Part model, mm, in its own coordinate system. A direction names the side the tool comes from. Give positions to 0.01 mm unless a question says otherwise; leave off trailing zeros. Write each loop counter-clockwise with the first axis right and the second up, starting at its lowest first coordinate (ties: lowest second). Pieces come first, ordered by that corner, then holes. Notation, with made-up numbers: (52, 4.25) - (73, 4.25) arc R20 ccw to (73, 40.25) - close; hole circle Ø8 at (44.25, 29.25). An arc over 180 degrees is marked (long way). Answer in a Markdown table with one row per item. Add a question column.
1. Band-saw the part on B-B on x = 24.5. Write the cut outline in (y, z), plus the area to 3 significant figures.
2. Band-saw the part on D-D on x = 0. Write the cut outline in (y, z), plus the area to 4 significant figures.
3. Band-saw the part on A-A on z = 5. Write the cut outline in (x, y).
4. Probe line 1 along X through (y, z) = (10.75, 5); line 2 along Y through (x, z) = (-7.5, 85.5); line 3 along X through (y, z) = (8.5, 65). List the from-to ranges inside material, lowest first.
5. Band-saw the part on C-C on y = -6.5. Write the cut outline in (x, z).
6. Which spindle directions (+Z, -Z, +X, -X, +Y, -Y) get a long thin tool onto all of the face, cutting with end or side? Do faces 5 (the flat face through (19, -1, 54)), 6 (the cylindrical face through (-15.58, -12.39, 54.23)). Say none if no direction does.
7. Drop flat-ended pins along their axis: pin 1 Ø3.5 at (x, z) = (24.5, 25) entering from -Y; pin 2 Ø3.5 at (x, z) = (-23.5, 62.5) entering from -Y; pin 3 Ø10 at (x, z) = (21, 52) entering from -Y; pin 4 Ø1 at (x, z) = (-13, 50) entering from -Y. Give the stop position or say it passes through.
8. Pull direction Z, two halves, no side cores. Call faces 1 (the cylindrical face through (24, 9, 103)), 2 (the flat face through (-25, 3, 54)), 3 (the flat face through (0, 11, 110)), 4 (the cylindrical face through (-25, 9, 43)): released by +Z, released by -Z, zero draft, split by the parting line, or undercut.
```python
from build123d import *

# Parameters (mm, degrees)
CROQUIS1_R              = 10.25
SALIENTE_EXTRUIR1_DEPTH = 110
CORTAR_EXTRUIR1_REACH   = 117.59
CROQUIS2_R              = 2.06


with BuildPart() as part:
    # Croquis1 → Saliente-Extruir1 (new body)
    with BuildSketch(Plane.XY):
        with BuildLine():
            Line((30, 16), (-30, 16))
            Line((-30, 16), (-30, 3))
            Line((-30, 3), (-19, 3))
            Line((-19, 3), (-19, -4))
            ThreePointArc((-19, -4), (-15.485281374, -12.485281374), (-7, -16))
            Line((-7, -16), (7, -16))
            ThreePointArc((7, -16), (15.485281374, -12.485281374), (19, -4))
            Line((19, -4), (19, 3))
            Line((19, 3), (30, 3))
            Line((30, 3), (30, 16))
        make_face()
        Circle(CROQUIS1_R, mode=Mode.SUBTRACT)
    extrude(amount=SALIENTE_EXTRUIR1_DEPTH)

    # Croquis2 → Cortar-Extruir1 (cut, up to next)
    with BuildSketch(Plane.XZ.offset(-3), mode=Mode.PRIVATE) as cortar_extruir1_sk1:
        with Locations(Location((-24.5, 105, 0), (0, 0, 270))):
            Circle(CROQUIS2_R)
    cortar_extruir1_tool1 = extrude(cortar_extruir1_sk1.sketch, amount=-CORTAR_EXTRUIR1_REACH, mode=Mode.PRIVATE) & part.part
    # Croquis2 → Cortar-Extruir1 (cut, up to next)
    with BuildSketch(Plane.XZ.offset(-3), mode=Mode.PRIVATE) as cortar_extruir1_sk2:
        with Locations(Location((-24.5, 85, 0), (0, 0, 270))):
            Circle(CROQUIS2_R)
    cortar_extruir1_tool2 = extrude(cortar_extruir1_sk2.sketch, amount=-CORTAR_EXTRUIR1_REACH, mode=Mode.PRIVATE) & part.part
    # Croquis2 → Cortar-Extruir1 (cut, up to next)
    with BuildSketch(Plane.XZ.offset(-3), mode=Mode.PRIVATE) as cortar_extruir1_sk3:
        with Locations(Location((-24.5, 65, 0), (0, 0, 270))):
            Circle(CROQUIS2_R)
    cortar_extruir1_tool3 = extrude(cortar_extruir1_sk3.sketch, amount=-CORTAR_EXTRUIR1_REACH, mode=Mode.PRIVATE) & part.part
    # Croquis2 → Cortar-Extruir1 (cut, up to next)
    with BuildSketch(Plane.XZ.offset(-3), mode=Mode.PRIVATE) as cortar_extruir1_sk4:
        with Locations(Location((-24.5, 45, 0), (0, 0, 270))):
            Circle(CROQUIS2_R)
    cortar_extruir1_tool4 = extrude(cortar_extruir1_sk4.sketch, amount=-CORTAR_EXTRUIR1_REACH, mode=Mode.PRIVATE) & part.part
    # Croquis2 → Cortar-Extruir1 (cut, up to next)
    with BuildSketch(Plane.XZ.offset(-3), mode=Mode.PRIVATE) as cortar_extruir1_sk5:
        with Locations(Location((-24.5, 25, 0), (0, 0, 270))):
            Circle(CROQUIS2_R)
    cortar_extruir1_tool5 = extrude(cortar_extruir1_sk5.sketch, amount=-CORTAR_EXTRUIR1_REACH, mode=Mode.PRIVATE) & part.part
    # Croquis2 → Cortar-Extruir1 (cut, up to next)
    with BuildSketch(Plane.XZ.offset(-3), mode=Mode.PRIVATE) as cortar_extruir1_sk6:
        with Locations(Location((-24.5, 5, 0), (0, 0, 270))):
            Circle(CROQUIS2_R)
    cortar_extruir1_tool6 = extrude(cortar_extruir1_sk6.sketch, amount=-CORTAR_EXTRUIR1_REACH, mode=Mode.PRIVATE) & part.part
    # Croquis2 → Cortar-Extruir1 (cut, up to next)
    with BuildSketch(Plane.XZ.offset(-3), mode=Mode.PRIVATE) as cortar_extruir1_sk7:
        with Locations(Location((24.5, 5, 0), (0, 0, 270))):
            Circle(CROQUIS2_R)
    cortar_extruir1_tool7 = extrude(cortar_extruir1_sk7.sketch, amount=-CORTAR_EXTRUIR1_REACH, mode=Mode.PRIVATE) & part.part
    # Croquis2 → Cortar-Extruir1 (cut, up to next)
    with BuildSketch(Plane.XZ.offset(-3), mode=Mode.PRIVATE) as cortar_extruir1_sk8:
        with Locations(Location((24.5, 25, 0), (0, 0, 270))):
            Circle(CROQUIS2_R)
    cortar_extruir1_tool8 = extrude(cortar_extruir1_sk8.sketch, amount=-CORTAR_EXTRUIR1_REACH, mode=Mode.PRIVATE) & part.part
    # Croquis2 → Cortar-Extruir1 (cut, up to next)
    with BuildSketch(Plane.XZ.offset(-3), mode=Mode.PRIVATE) as cortar_extruir1_sk9:
        with Locations(Location((24.5, 45, 0), (0, 0, 270))):
            Circle(CROQUIS2_R)
    cortar_extruir1_tool9 = extrude(cortar_extruir1_sk9.sketch, amount=-CORTAR_EXTRUIR1_REACH, mode=Mode.PRIVATE) & part.part
    # Croquis2 → Cortar-Extruir1 (cut, up to next)
    with BuildSketch(Plane.XZ.offset(-3), mode=Mode.PRIVATE) as cortar_extruir1_sk10:
        with Locations(Location((24.5, 65, 0), (0, 0, 270))):
            Circle(CROQUIS2_R)
    cortar_extruir1_tool10 = extrude(cortar_extruir1_sk10.sketch, amount=-CORTAR_EXTRUIR1_REACH, mode=Mode.PRIVATE) & part.part
    # Croquis2 → Cortar-Extruir1 (cut, up to next)
    with BuildSketch(Plane.XZ.offset(-3), mode=Mode.PRIVATE) as cortar_extruir1_sk11:
        with Locations(Location((24.5, 85, 0), (0, 0, 270))):
            Circle(CROQUIS2_R)
    cortar_extruir1_tool11 = extrude(cortar_extruir1_sk11.sketch, amount=-CORTAR_EXTRUIR1_REACH, mode=Mode.PRIVATE) & part.part
    # Croquis2 → Cortar-Extruir1 (cut, up to next)
    with BuildSketch(Plane.XZ.offset(-3), mode=Mode.PRIVATE) as cortar_extruir1_sk12:
        with Locations(Location((24.5, 105, 0), (0, 0, 270))):
            Circle(CROQUIS2_R)
    cortar_extruir1_tool12 = extrude(cortar_extruir1_sk12.sketch, amount=-CORTAR_EXTRUIR1_REACH, mode=Mode.PRIVATE) & part.part
    add(cortar_extruir1_tool1.solids().sort_by_distance((-24.5, 3, 105))[0], mode=Mode.SUBTRACT)
    add(cortar_extruir1_tool2.solids().sort_by_distance((-24.5, 3, 85))[0], mode=Mode.SUBTRACT)
    add(cortar_extruir1_tool3.solids().sort_by_distance((-24.5, 3, 65))[0], mode=Mode.SUBTRACT)
    add(cortar_extruir1_tool4.solids().sort_by_distance((-24.5, 3, 45))[0], mode=Mode.SUBTRACT)
    add(cortar_extruir1_tool5.solids().sort_by_distance((-24.5, 3, 25))[0], mode=Mode.SUBTRACT)
    add(cortar_extruir1_tool6.solids().sort_by_distance((-24.5, 3, 5))[0], mode=Mode.SUBTRACT)
    add(cortar_extruir1_tool7.solids().sort_by_distance((24.5, 3, 5))[0], mode=Mode.SUBTRACT)
    add(cortar_extruir1_tool8.solids().sort_by_distance((24.5, 3, 25))[0], mode=Mode.SUBTRACT)
    add(cortar_extruir1_tool9.solids().sort_by_distance((24.5, 3, 45))[0], mode=Mode.SUBTRACT)
    add(cortar_extruir1_tool10.solids().sort_by_distance((24.5, 3, 65))[0], mode=Mode.SUBTRACT)
    add(cortar_extruir1_tool11.solids().sort_by_distance((24.5, 3, 85))[0], mode=Mode.SUBTRACT)
    add(cortar_extruir1_tool12.solids().sort_by_distance((24.5, 3, 105))[0], mode=Mode.SUBTRACT)


solid = part.part
```
Values:
| question | item | result |
|---|---|---|
| 1 | outline | (3, 0) - (16, 0) - (16, 2.94) - (3, 2.94) - close; (3, 7.06) - (16, 7.06) - (16, 22.94) - (3, 22.94) - close; (3, 27.06) - (16, 27.06) - (16, 42.94) - (3, 42.94) - close; (3, 47.06) - (16, 47.06) - (16, 62.94) - (3, 62.94) - close; (3, 67.06) - (16, 67.06) - (16, 82.94) - (3, 82.94) - close; (3, 87.06) - (16, 87.06) - (16, 102.94) - (3, 102.94) - close; (3, 107.06) - (16, 107.06) - (16, 110) - (3, 110) - close |
| 1 | area | 1,110 mm² |
| 2 | outline | (-16, 0) - (-10.25, 0) - (-10.25, 110) - (-16, 110) - close; (10.25, 0) - (16, 0) - (16, 110) - (10.25, 110) - close |
| 2 | area | 1,265 mm² |
| 3 | outline | (-30, 3) - (-26.56, 3) - (-26.56, 16) - (-30, 16) - close; (-22.44, 3) - (-19, 3) - (-19, -4) arc R12 ccw to (-7, -16) - (7, -16) arc R12 ccw to (19, -4) - (19, 3) - (22.44, 3) - (22.44, 16) - (-22.44, 16) - close; (26.56, 3) - (30, 3) - (30, 16) - (26.56, 16) - close; hole circle Ø20.5 at (0, 0) |
| 4 | line 1 | x = -30 to -26.56, -22.44 to 22.44, 26.56 to 30 |
| 4 | line 2 | y = -15.99 to -6.99, 6.99 to 16 |
| 4 | line 3 | x = -30 to -26.56, -22.44 to -5.73, 5.73 to 22.44, 26.56 to 30 |
| 5 | outline | (-18.74, 0) - (-7.93, 0) - (-7.93, 110) - (-18.74, 110) - close; (7.93, 0) - (18.74, 0) - (18.74, 110) - (7.93, 110) - close |
| 6 | face 5 | +Z, -Z, +X, -Y |
| 6 | face 6 | +Z, -Z, -X, -Y |
| 7 | pin 1 | passes through |
| 7 | pin 2 | stops at y = 3 |
| 7 | pin 3 | stops at y = -11.94 |
| 7 | pin 4 | stops at y = -14.67 |
| 8 | face 1 | undercut |
| 8 | face 2 | zero draft |
| 8 | face 3 | released by +Z |
| 8 | face 4 | undercut |
